```python
from build123d import *

# Parameters (mm, degrees)
F1_DEPTH      = 31.75
F2_W          = 14.5460739732
F2_H          = 83.8538557291
F3_DEPTH      = 114.301
F3_DEPTH_BACK = 114.301
F4_R          = 3.175
F5_T          = 2.54
F5_T3_DEPTH   = 215.6340543381


# Not quite as in the source:
# - a shell that OpenCascade refuses in one call is made with other operations: the cavity is built on its own and cut out


with BuildPart() as f1:
    # F0 (on Front) → F1 (new body, symmetric)
    with BuildSketch(Plane.XZ):
        with BuildLine():
            Line((-114.3, 0), (114.3, 0))
            ThreePointArc((114.3, 0), (0, 114.3), (-114.3, 0))
        make_face()
    extrude(amount=F1_DEPTH, both=True)

    # F2 (on Right) → F3 (cut, two sides)
    with BuildSketch(Plane.YZ) as f3_sk:
        with Locations((1.2597227469, 86.4380225539)):
            Rectangle(F2_W, F2_H)
    extrude(amount=-F3_DEPTH, mode=Mode.SUBTRACT)
    extrude(f3_sk.sketch, amount=F3_DEPTH_BACK, mode=Mode.SUBTRACT)

    # F4
    f4_edges = [f1.edges().sort_by_distance(p)[0] for p in [
        (0, 31.75, 114.3),
        (0, -31.75, 114.3),
    ]]
    fillet(f4_edges, radius=F4_R)

    # F5: shell of thickness 2.54, made by hand


with BuildPart() as f5_core1:
    # F5_t2: copy of F1
    add(f1.part)

    # the walls: a layer under each face that stays
    f5_faces = [f5_core1.faces().sort_by_distance(p)[0] for p in [
        (0, 31.75, 55.5625),
        (0, 30.8200640303, 113.3700640303),
        (98.9867036526, 19.05, 57.15),
        (0, -30.8200640303, 113.3700640303),
        (0, -31.75, 55.5625),
        (0, 8.5327597335, 79.4055473447),
        (0, 1.2597227469, 44.5110946894),
        (0, -6.0133142397, 79.4055473447),
    ]]
    thicken(f5_faces, amount=-F5_T, mode=Mode.SUBTRACT)

    # F5_s4 → F5_t3 (cut)
    with BuildSketch(Plane.YZ.offset(-107.8170271691)):
        Polygon((8.5073597335, 44.5364946894), (11.0727597335, 44.5110946894), (11.0727597335, 41.9710946894), (8.5327597335, 41.9710946894), align=None)
        Polygon((-5.9879142397, 44.5364946894), (-6.0133142397, 41.9710946894), (-8.5533142397, 41.9710946894), (-8.5533142397, 44.5110946894), align=None)
    extrude(amount=F5_T3_DEPTH, mode=Mode.SUBTRACT)


with BuildPart() as f1_1:
    add(f1.part)

    # what is left inside the walls is the cavity
    f5_cavity = [f5_core1.part.solids().sort_by_distance(p)[0] for p in [
        (0, 29.1846, 37.041667),
    ]]
    add(f5_cavity, mode=Mode.SUBTRACT)


solid = f1_1.part
```
The listing builds one solid part. Answer for the finished solid, in the listing's coordinates (mm). A direction names the side the tool comes from. Round coordinates to 2 decimals unless told otherwise and drop trailing zeros. Loops run counter-clockwise (first coordinate to the right, second up) from the corner with the lowest first, then second, coordinate; pieces in that order, holes last.
Q1. Find the intervals of material crossed by line 1 (Y direction, x = 65, z = 90); line 2 (Y direction, x = -29.5, z = 5); line 3 (X direction, y = -20, z = 38.5), in increasing order.
Q2. Section B-B, the plane z = 64.5 is taken. Count the separate pieces of the cut face and the enclosed holes in it, then the cut area to 3 significant figures.
Q3. Which of the six approach directions +Z, -Z, +X, -X, +Y, -Y give full straight-line access (tool end or side, diameter ignored) to faces 1 (the face through (1, 8.533, 71)), 2 (the face through (1, 1, 41.971)), 3 (the face through (-1, -31, 0))?
Q4. For a pull along X with two mould halves and no side action, classify faces 4 (the face through (-2, 31.75, 44)), 5 (the face through (-2, 29.21, 44)), 6 (the face through (2.513, -6.75, 114.272)) as released by +X, released by -X, zero draft, split by the parting line, or undercut.
Q5. Section C-C, the plane y = -25 is taken. Determine the outline of the cut face in (x, z), then the cut area to 3 significant figures.
Q6. Section A-A, the plane x = 0 is taken. Determine the outline of the cut face in (y, z) (3 decimals), then the cut area to 3 significant figures.
Q7. Given pin 1 Ø4 at (y, z) = (7.5, 94) entering from +X; pin 2 Ø4.5 at (x, y) = (44.5, 1) entering from +Z; pin 3 Ø10 at (x, y) = (-41.5, 16) entering from -Z, each flat-ended and moving along its own axis, determine where each tip first touches the part or whether it passes through.
Completed:
1. line 1: y = -31.75 to -29.21, -8.55 to -6.01, 8.53 to 11.07, 29.21 to 31.75
1. line 2: y = -31.75 to -29.21, 29.21 to 31.75
1. line 3: x = -107.62 to -104.92, 104.92 to 107.62
2. separate pieces: 2
2. enclosed holes: 2
2. area: 2,150 mm2
3. face 1: +Z, +X, -X
3. face 2: -Z
3. face 3: -Z, +X, -X, +Y, -Y
4. face 4: zero draft
4. face 5: undercut
4. face 6: split by the parting line
5. outline: (-114.3, 0) - (-111.76, 0) arc R111.76 cw to (111.76, 0) - (114.3, 0) arc R114.3 ccw to start
5. area: 902 mm2
6. outline: (-31.75, 0) - (-29.21, 0) - (-29.21, 111.125) arc R0.635 cw to (-28.575, 111.76) - (-8.553, 111.76) - (-8.553, 41.971) - (11.073, 41.971) - (11.073, 111.76) - (28.575, 111.76) arc R0.635 cw to (29.21, 111.125) - (29.21, 0) - (31.75, 0) - (31.75, 111.125) arc R3.175 ccw to (28.575, 114.3) - (8.533, 114.3) - (8.533, 44.511) - (-6.013, 44.511) - (-6.013, 114.3) - (-28.575, 114.3) arc R3.175 ccw to (-31.75, 111.125) - close
6. area: 1,080 mm2
7. pin 1: stops at x = 67.44
7. pin 2: stops at z = 44.51
7. pin 3: stops at z = 41.97
